Verification items for the finished model (mm, model axes). Face numbers are marked on the shaded views. Give positions to 0.01 mm unless a question says otherwise; leave off trailing zeros. Write each loop counter-clockwise with the first axis right and the second up, starting at its lowest first coordinate (ties: lowest second). Pieces come first, ordered by that corner, then holes. Notation, with made-up numbers: (0, 83) -> (32, 83) arc R22 cw to (32, 96) -> close; hole circle Ø7 at (60.5, 60.5). An arc over 180 degrees is marked (long way). Use one line per item in the form item = value. Start each with the question number.
(1) Section check A-A, the plane y = 0. Record the cut outline in (x, z), plus the area to 3 significant figures.
(2) Release check for a two-part mould opening along Y. For the marked faces 1, 2, 3 and 4 record: pulls with the +Y half, pulls with the -Y half, needs draft (parallel to the pull), parting line crosses it, or undercut.
(3) Scan lines: L1, parallel to Y at x = 0, z = -0.25; L2, parallel to Y at x = 16.5, z = -1.3; L3, parallel to Y at x = 4, z = -1.05. Record each from-to range of solid material in increasing order.
(4) Section check C-C, the plane x = 0. Record the cut outline in (y, z), plus the area to 3 significant figures.
(5) Section check D-D, the plane z = 0.3. State how many separate pieces and enclosed holes the cut face has, plus the area to 3 significant figures.
(6) Depth check by flat-ended pin: pin 1 Ø1 at (x, z) = (-11, 1) entering from -Y; pin 2 Ø0.8 at (x, z) = (16, 0) entering from -Y; pin 3 Ø0.8 at (y, z) = (14.5, 0.5) entering from +X. Enter the tip coordinate at first touch or a pass-through.
(7) Section check B-B, the plane x = -6. Record the cut outline in (y, z), plus the area to 3 significant figures.
from build123d import *

# Parameters (mm, degrees)
SKETCH_1_R      = 8.05
SKETCH_1_W      = 10
SKETCH_1_H      = 2.8
EXTRUDE_1_DEPTH = 1.4
FILLET_1_R      = 5


with BuildPart() as part:
    # Эскиз1 → Бобышка-Вытянуть1 (new, symmetric)
    with BuildSketch(Plane.XY):
        Polygon((-15, 12.6), (-17.8, 12.6), (-17.8, 7.6), (-15, 7.6), (-15, -7.6), (-17.8, -7.6), (-17.8, -12.6), (-15, -12.6), (-15, -18), (15, -18), (15, -12.6), (17.8, -12.6), (17.8, -7.6), (15, -7.6), (15, 7.6), (17.8, 7.6), (17.8, 12.6), (15, 12.6), (12, 12.6), (12, 15.4), (15, 15.4), (15, 18), (8, 18), (8, 15.2), (-8, 15.2), (-8, 18), (-15, 18), (-15, 15.4), (-12, 15.4), (-12, 12.6), align=None)
        Circle(SKETCH_1_R, mode=Mode.SUBTRACT)
        with Locations((0, -14)):
            Rectangle(SKETCH_1_W, SKETCH_1_H, mode=Mode.SUBTRACT)
    extrude(amount=EXTRUDE_1_DEPTH, both=True)

    # Скругление1
    # the kernel refuses this fillet: 5 mm, written as the material it takes off along each edge
    with BuildSketch(Plane(origin=(15, 18, -12.3658561), x_dir=(-1, 0, 0), z_dir=(0, 0, 1))) as fillet_1_piece_1:
        with BuildLine():
            CenterArc((4.38634244, 5), FILLET_1_R, 208.685402014, 61.314597986)
            Line((0, 2.6), (-0.087726849, 2.552))
            ThreePointArc((-0.087726849, 2.552), (-0.1, 1.3), (-0.1, 0))
            Line((-0.1, 0), (0, -0.1))
            Line((0, -0.1), (4.38634244, -0.1))
            Line((4.38634244, -0.1), (4.38634244, 0))
        make_face()
    extrude(amount=24.731712199, mode=Mode.SUBTRACT)
    with BuildSketch(Plane(origin=(15, -18, -13.9), x_dir=(0, 1, 0), z_dir=(0, 0, 1)), Plane(origin=(-15, -18, -13.9), x_dir=(1, 0, 0), z_dir=(0, 0, 1))) as fillet_1_piece_2:
        with BuildLine():
            CenterArc((FILLET_1_R, FILLET_1_R), FILLET_1_R, 180, 90)
            Line((0, FILLET_1_R), (-FILLET_1_R * 0.02, FILLET_1_R))
            Line((-FILLET_1_R * 0.02, FILLET_1_R), (-FILLET_1_R * 0.02, -FILLET_1_R * 0.02))
            Line((-FILLET_1_R * 0.02, -FILLET_1_R * 0.02), (FILLET_1_R, -FILLET_1_R * 0.02))
            Line((FILLET_1_R, -FILLET_1_R * 0.02), (FILLET_1_R, 0))
        make_face()
    extrude(amount=27.8, mode=Mode.SUBTRACT)
    with BuildSketch(Plane(origin=(-15, 18, -12.3658561), x_dir=(0, -1, 0), z_dir=(0, 0, 1))) as fillet_1_piece_3:
        with BuildLine():
            CenterArc((5, 4.38634244), FILLET_1_R, 180, 61.314597986)
            Line((0, 4.38634244), (-0.1, 4.38634244))
            Line((-0.1, 4.38634244), (-0.1, 0))
            Line((-0.1, 0), (0, -0.1))
            ThreePointArc((0, -0.1), (1.3, -0.1), (2.552, -0.087726849))
            Line((2.552, -0.087726849), (2.6, 0))
        make_face()
    extrude(amount=24.731712199, mode=Mode.SUBTRACT)


solid = part.part
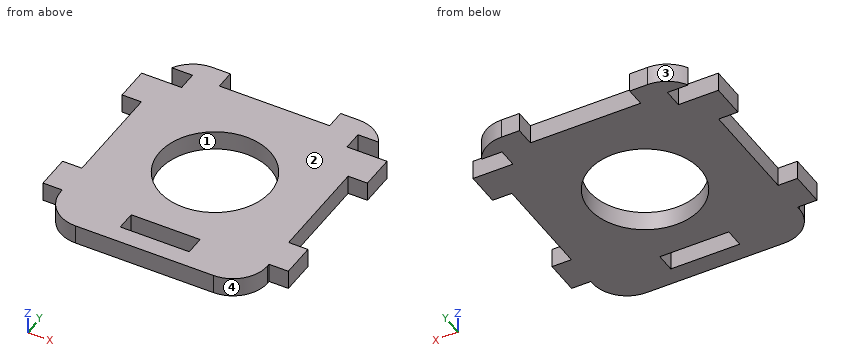
Completed:
q1.outline = (-15, -1.4) -> (-8.05, -1.4) -> (-8.05, 1.4) -> (-15, 1.4) -> close; (8.05, -1.4) -> (15, -1.4) -> (15, 1.4) -> (8.05, 1.4) -> close
q1.area = 38.9 mm²
q2.face_1 = undercut
q2.face_2 = needs draft
q2.face_3 = pulls with the +Y half
q2.face_4 = pulls with the -Y half
q3.L1 = -18 to -15.4, -12.6 to -8.05, 8.05 to 15.2
q3.L2 = -12.6 to -7.6, 7.6 to 12.6
q3.L3 = -18 to -15.4, -12.6 to -6.99, 6.99 to 15.2
q4.outline = (-18, -1.4) -> (-15.4, -1.4) -> (-15.4, 1.4) -> (-18, 1.4) -> close; (-12.6, -1.4) -> (-8.05, -1.4) -> (-8.05, 1.4) -> (-12.6, 1.4) -> close; (8.05, -1.4) -> (15.2, -1.4) -> (15.2, 1.4) -> (8.05, 1.4) -> close
q4.area = 40.0 mm²
q5.separate_pieces = 1
q5.enclosed_holes = 2
q5.area = 826 mm²
q6.pin_1 = -17.97
q6.pin_2 = -12.6
q6.pin_3 = 12
q7.outline = (-18, -1.4) -> (-5.37, -1.4) -> (-5.37, 1.4) -> (-18, 1.4) -> close; (5.37, -1.4) -> (15.2, -1.4) -> (15.2, 1.4) -> (5.37, 1.4) -> close
q7.area = 62.9 mm²
